Work out the finished part from the listing and answer in its coordinate system (mm). A direction names the side the tool comes from. Round coordinates to 2 decimals unless told otherwise and drop trailing zeros. Write each loop counter-clockwise with the first axis right and the second up, starting at its lowest first coordinate (ties: lowest second). Pieces come first, ordered by that corner, then holes.
1. Straight lines are drawn through the part: probe 1 along X at (y, z) = (-19, -4.45); probe 2 along X at (y, z) = (112, -4.7); probe 3 along Y at (x, z) = (-2, -3.1). For each, find the intervals that lie inside material, in ascending order.
2. Find section A-A (y = 112). Write down the section's boundary in (x, z), and give its area (3 significant figures).
3. Find section B-B (y = 65). Write down the section's boundary in (x, z), and give its area (3 significant figures).
4. Flat-ended cylindrical pins translate along their axes: pin 1 Ø4.5 at (x, y) = (6.5, 6.5) entering from -Z; pin 2 Ø1 at (x, z) = (-20, -3.5) entering from -Y; pin 3 Ø2.5 at (y, z) = (78, -4.5) entering from -X; pin 4 Ø8 at (x, y) = (4, 54) entering from -Z. Find the tip coordinate at first contact, or state that the pin passes through.
5. A tool of negligible diameter and unlimited length cuts with its end or side. For faces 5 (the face through (1.15, 31.37, -0.49)), 6 (the face through (-25.894, -3.509, -3.465)), 7 (the face through (0.25, -21, -3)), 8 (the face through (-15.7, 2.75, -0.8)), from which of +Z, -Z, +X, -X, +Y, -Y can it reach the whole face along a straight path? Write none if from no direction.
6. Find section D-D (y = 28). Write down the section's boundary in (x, z), and give its area (3 significant figures).
7. Determine the mould class of faces 1 (the face through (-2.646, 111.787, -3.465)), 2 (the face through (-8.054, -0.785, -3.465)), 3 (the face through (-2.75, -28.37, -2.96)), 4 (the face through (-4.787, 0.191, -0.493)) for opening direction Y: pulls with the +Y half, pulls with the -Y half, needs draft (parallel to the pull), parting line crosses it, or undercut.
8. Find section C-C (z = -3.2). Count the separate pieces of the cut face and the enclosed holes in it, and give its area (3 significant figures).
```python
from build123d import *

# Parameters (mm, degrees)
F0_R     = 4
F0_W     = 19
F0_H     = 69
F1_DEPTH = 1
F2_R     = 5.9
F2_R_2   = 4
F3_DEPTH = 5
F5_DEPTH = 2.02602933
F6_W     = 5
F6_H     = 132.25
F7_DEPTH = 5
F8_W     = 2.5
F8_H     = 20
F9_DEPTH = 6


with BuildPart() as f1:
    # F0 (on Top) → F1 (new body)
    with BuildSketch(Plane.XY):
        with BuildLine():
            ThreePointArc((2.2980970389, 2.2980970389), (3.0026084807, 1.2437211552), (3.25, 0))
            ThreePointArc((3.25, 0), (1.2437211552, -3.0026084807), (-2.2980970389, -2.2980970389))
            Line((-2.2980970389, -2.2980970389), (-7.3461940777, 2.75))
            Line((-7.3461940777, 2.75), (-29, 2.75))
            Line((-29, 2.75), (-29, -11.25))
            Line((-29, -11.25), (13.25, -11.25))
            Line((13.25, -11.25), (13.25, 52))
            Line((13.25, 52), (-5.75, 52))
            Line((-5.75, 52), (-5.75, 38.2720779386))
            Line((-5.75, 38.2720779386), (8.25, 24.2720779386))
            Line((8.25, 24.2720779386), (8.25, 11.7855339059))
            Line((8.25, 11.7855339059), (0.5303300859, 4.0658639918))
            Line((0.5303300859, 4.0658639918), (2.2980970389, 2.2980970389))
        make_face()
        with Locations((-20, -3.25)):
            Circle(F0_R, mode=Mode.SUBTRACT)
        with Locations((3.25, 42)):
            Circle(F0_R, mode=Mode.SUBTRACT)
        with Locations((3.75, 86.5)):
            Rectangle(F0_W, F0_H)
        with Locations((3.25, 112)):
            Circle(F0_R, mode=Mode.SUBTRACT)
    extrude(amount=-F1_DEPTH)

    # F2 (on face) → F3 (join)
    with BuildSketch(Plane(origin=(0, 0, -1), x_dir=(1, 0, 0), z_dir=(0, 0, -1))):
        with Locations((-20, 3.25)):
            Circle(F2_R)
        with Locations((-20, 3.25)):
            Circle(F2_R_2, mode=Mode.SUBTRACT)
        with BuildLine():
            Line((-11.5888347648, -2.75), (-8.2554414615, 0.5833933033))
            ThreePointArc((-8.2554414615, 0.5833933033), (-7.5296004881, 3.434789362), (-5.8520364605, 5.8520364605))
            Line((-5.8520364605, 5.8520364605), (-14.4540729211, -2.75))
            Line((-14.4540729211, -2.75), (-11.5888347648, -2.75))
        make_face()
        with BuildLine():
            ThreePointArc((-4.4194173824, 4.4194173824), (2.3917714523, 5.7742470782), (6.25, 0))
            ThreePointArc((6.25, 0), (5.7742470782, -2.3917714523), (4.4194173824, -4.4194173824))
            Line((4.4194173824, -4.4194173824), (2.6516504294, -6.1871843354))
            Line((2.6516504294, -6.1871843354), (3.8108825911, -7.346416497))
            ThreePointArc((3.8108825911, -7.346416497), (4.8888949746, -6.6776767965), (5.8520364605, -5.8520364605))
            ThreePointArc((5.8520364605, -5.8520364605), (7.6460541085, -3.1670993104), (8.27602933, 0))
            ThreePointArc((8.27602933, 0), (3.1670993104, 7.6460541085), (-5.8520364605, 5.8520364605))
            ThreePointArc((-5.8520364605, 5.8520364605), (-7.5296004881, 3.434789362), (-8.2554414615, 0.5833933033))
            Line((-8.2554414615, 0.5833933033), (-4.4194173824, 4.4194173824))
        make_face()
        with BuildLine():
            ThreePointArc((5.8520364605, -5.8520364605), (4.8888949746, -6.6776767965), (3.8108825911, -7.346416497))
            Line((3.8108825911, -7.346416497), (4.0842695076, -7.6198034135))
            Line((4.0842695076, -7.6198034135), (5.8520364605, -5.8520364605))
        make_face()
        with Locations((3.25, -42)):
            Circle(F2_R)
        with Locations((3.25, -42)):
            Circle(F2_R_2, mode=Mode.SUBTRACT)
        with Locations((3.25, -112)):
            Circle(F2_R)
        with Locations((3.25, -112)):
            Circle(F2_R_2, mode=Mode.SUBTRACT)
    extrude(amount=F3_DEPTH)

    # F4 (on face) → F5 (join, through all)
    with BuildSketch(Plane(origin=(5.8520364605, 5.8520364605, 0), x_dir=(-0.7071067812, 0.7071067812, 0), z_dir=(0.7071067812, 0.7071067812, 0))):
        Polygon((2.5, -1), (2.5, -6), (7, -6), (7, -5.5), align=None)
    extrude(amount=-F5_DEPTH)

    # F6 (on face) → F7 (join)
    with BuildSketch(Plane(origin=(0, 0, -1), x_dir=(1, 0, 0), z_dir=(0, 0, -1))):
        with Locations((10.75, -54.875)):
            Rectangle(F6_W, F6_H)
    extrude(amount=F7_DEPTH)

    # F8 (on Top) → F9 (join)
    with BuildSketch(Plane.XY):
        Polygon((11.25, -11.25), (13.25, -11.25), (13.25, -6.25), (5.4249572783, -6.25), (-3.25, -6.25), (-3.25, -8.4540729211), (-3.25, -11.25), (-1.25, -11.25), (0.25, -11.25), (3.75, -11.25), (6.25, -11.25), (9.75, -11.25), align=None)
        with BuildLine():
            Line((11.25, -21.25), (11.25, -11.25))
            Line((11.25, -11.25), (9.75, -11.25))
            Line((9.75, -11.25), (9.75, -31.25))
            Line((9.75, -31.25), (11.25, -31.25))
            ThreePointArc((11.25, -31.25), (12.7368329805, -28.4122776602), (13.25, -25.25))
            Line((13.25, -25.25), (13.25, -21.25))
            Line((13.25, -21.25), (11.25, -21.25))
        make_face()
        with BuildLine():
            Line((5.4249572783, -6.25), (13.25, -6.25))
            Line((13.25, -6.25), (13.25, 0))
            Line((13.25, 0), (8.27602933, 0))
            ThreePointArc((8.27602933, 0), (7.5296004881, -3.434789362), (5.4249572783, -6.25))
        make_face()
        with Locations((5, -21.25)):
            Rectangle(F8_W, F8_H)
        Polygon((-3.25, -8.4540729211), (-3.25, -6.25), (-5.8520364605, -5.8520364605), align=None)
        with BuildLine():
            Line((0.25, -31.25), (0.25, -11.25))
            Line((0.25, -11.25), (-1.25, -11.25))
            Line((-1.25, -11.25), (-1.25, -21.25))
            Line((-1.25, -21.25), (-3.25, -21.25))
            Line((-3.25, -21.25), (-3.25, -25.25))
            ThreePointArc((-3.25, -25.25), (-2.7368329805, -28.4122776602), (-1.25, -31.25))
            Line((-1.25, -31.25), (0.25, -31.25))
        make_face()
    extrude(amount=-F9_DEPTH)


solid = f1.part
```
Worked answers:
1. probe 1: x = -1.25 to 0.25, 3.75 to 6.25, 9.75 to 11.25
1. probe 2: x = -2.65 to -0.75, 7.25 to 13.25
1. probe 3: y = -30.09 to -21.25, -11.25 to -5.92, 39.31 to 44.69, 109.31 to 114.69
2. outline: (-5.75, -1) - (-2.65, -1) - (-2.65, -6) - (-0.75, -6) - (-0.75, 0) - (-5.75, 0) - close; (7.25, -6) - (13.25, -6) - (13.25, 0) - (7.25, 0) - close
2. area: 50.5 mm2
3. outline: (-5.75, -1) - (8.25, -1) - (8.25, -6) - (13.25, -6) - (13.25, 0) - (-5.75, 0) - close
3. area: 44.0 mm2
4. pin 1: stops at z = -6
4. pin 2: stops at y = -9.15
4. pin 3: stops at x = 8.25
4. pin 4: stops at z = -1
5. face 5: +Z, -Z, -X
5. face 6: -Z
5. face 7: +Z, -Z, -Y
5. face 8: +Z, -Z, -X, +Y
6. outline: (4.52, -1) - (8.25, -1) - (8.25, -6) - (13.25, -6) - (13.25, 0) - (4.52, 0) - close
6. area: 33.7 mm2
7. face 1: undercut
7. face 2: pulls with the +Y half
7. face 3: pulls with the -Y half
7. face 4: undercut
8. separate pieces: 2
8. enclosed holes: 3
8. area: 1,100 mm2
